The model under review builds one solid part; all positions refer to its coordinate system, in mm. Face numbers are marked on the shaded views. A direction names the side the tool comes from. Coordinates: 2 decimals unless noted, no trailing zeros. Write each loop counter-clockwise with the first axis right and the second up, starting at its lowest first coordinate (ties: lowest second). Pieces come first, ordered by that corner, then holes.
1) Add section B-B, the plane x = 0.5. State the section outline as (y, z) points.
2) For P1, Ø1.4, axis at x = 0.5, y = 12.5, coming from the +Z side; P2, Ø1, axis at y = 23.5, z = 0.5, coming from the +X side; P3, Ø1, axis at y = 29, z = 0, coming from the -X side; P4, Ø3, axis at x = 0, y = 1, coming from the -Z side, all flat-tipped, find the tip position at first contact; note any pin that passes through.
3) Add section C-C, the plane y = 2.5. State the section outline as (x, z) points, then the cut area to 3 significant figures.
4) Add section A-A, the plane y = 27.5. State the section outline as (x, z) points, then the cut area to 3 significant figures.
5) For line 1 (X direction, y = 24, z = 0); line 2 (Z direction, x = 1.25, y = 11), list the stretches that pass through material, from the lowest coordinate up.
6) Add section D-D, the plane x = 3.5. State the section outline as (y, z) points, then the cut area to 3 significant figures.
7) Machinability: for the marked faces 1, 2, 3 and 4, which of the approach directions +Z, -Z, +X, -X, +Y, -Y give a long, thin tool a straight path to every point of the face, cutting with its end or side? Answer none if there is none.
from build123d import *

# Parameters (mm, degrees)
EXTRUDE_THIN1_DEPTH      = 30.4
EXTRUDE_THIN1_DEPTH_BACK = 1.6
EXTRUDE_THIN2_DEPTH      = 12
EXTRUDE_THIN3_DEPTH      = 1


with BuildPart() as part:
    # Sketch1 → Extrude-Thin1 (new body, two sides)
    with BuildSketch(Plane(origin=(0, 0, 0), x_dir=(1, 0, 0), z_dir=(0, 1, 0))) as extrude_thin1_sk:
        with BuildLine():
            Line((1.35, -0.6), (-1.35, -0.6))
            ThreePointArc((-1.35, -0.6), (-1.456066017, -0.556066017), (-1.5, -0.45))
            Line((-1.5, -0.45), (-1.5, 0.45))
            ThreePointArc((-1.5, 0.45), (-1.456066017, 0.556066017), (-1.35, 0.6))
            Line((-1.35, 0.6), (1.35, 0.6))
            ThreePointArc((1.35, 0.6), (1.456066017, 0.556066017), (1.5, 0.45))
            Line((1.5, 0.45), (1.5, -0.45))
            ThreePointArc((1.5, -0.45), (1.456066017, -0.556066017), (1.35, -0.6))
        make_face()
        with BuildLine():
            Line((1.35, -0.5), (-1.35, -0.5))
            ThreePointArc((-1.35, -0.5), (-1.385355339, -0.485355339), (-1.4, -0.45))
            Line((-1.4, -0.45), (-1.4, 0.45))
            ThreePointArc((-1.4, 0.45), (-1.385355339, 0.485355339), (-1.35, 0.5))
            Line((-1.35, 0.5), (1.35, 0.5))
            ThreePointArc((1.35, 0.5), (1.385355339, 0.485355339), (1.4, 0.45))
            Line((1.4, 0.45), (1.4, -0.45))
            ThreePointArc((1.4, -0.45), (1.385355339, -0.485355339), (1.35, -0.5))
        make_face(mode=Mode.SUBTRACT)
    extrude(amount=EXTRUDE_THIN1_DEPTH)
    extrude(extrude_thin1_sk.sketch, amount=-EXTRUDE_THIN1_DEPTH_BACK)

    # Sketch2 → Extrude-Thin2 (add, symmetric)
    with BuildSketch(Plane(origin=(0, 14, 0), x_dir=(-1, 0, 0), z_dir=(0, 1, 0))):
        with BuildLine():
            Line((-1.55, -0.45), (-1.55, 0.45))
            ThreePointArc((-1.55, 0.45), (-1.491421356, 0.591421356), (-1.35, 0.65))
            Line((-1.35, 0.65), (1.35, 0.65))
            ThreePointArc((1.35, 0.65), (1.491421356, 0.591421356), (1.55, 0.45))
            Line((1.55, 0.45), (1.55, -0.45))
            ThreePointArc((1.55, -0.45), (1.491421356, -0.591421356), (1.35, -0.65))
            Line((1.35, -0.65), (-1.35, -0.65))
            ThreePointArc((-1.35, -0.65), (-1.491421356, -0.591421356), (-1.55, -0.45))
        make_face()
        with BuildLine():
            Line((-1.5, -0.45), (-1.5, 0.45))
            ThreePointArc((-1.5, 0.45), (-1.456066017, 0.556066017), (-1.35, 0.6))
            Line((-1.35, 0.6), (1.35, 0.6))
            ThreePointArc((1.35, 0.6), (1.456066017, 0.556066017), (1.5, 0.45))
            Line((1.5, 0.45), (1.5, -0.45))
            ThreePointArc((1.5, -0.45), (1.456066017, -0.556066017), (1.35, -0.6))
            Line((1.35, -0.6), (-1.35, -0.6))
            ThreePointArc((-1.35, -0.6), (-1.456066017, -0.556066017), (-1.5, -0.45))
        make_face(mode=Mode.SUBTRACT)
    extrude(amount=EXTRUDE_THIN2_DEPTH, both=True)

    # Sketch3 → Extrude-Thin3 (add)
    with BuildSketch(Plane.XZ.offset(0.5)):
        with BuildLine():
            Line((0, 0.6), (-0.75, 0.6))
            ThreePointArc((-0.75, 0.6), (-1.043338791, 0.837132251), (-0.872943663, 1.173650974))
            ThreePointArc((-0.872943663, 1.173650974), (2.074168878, 1.680733699), (4.9, 0.702324945))
            Line((4.9, 0.702324945), (5.733615576, 0.149979879))
            Line((5.733615576, 0.149979879), (5.678381069, 0.066618321))
            Line((5.678381069, 0.066618321), (4.844765493, 0.618963387))
            ThreePointArc((4.844765493, 0.618963387), (2.066031557, 1.581065329), (-0.831962442, 1.082433983))
            ThreePointArc((-0.831962442, 1.082433983), (-0.945559194, 0.858088167), (-0.75, 0.7))
            Line((-0.75, 0.7), (0, 0.7))
            Line((0, 0.7), (0, 0.6))
        make_face()
    extrude(amount=EXTRUDE_THIN3_DEPTH)


solid = part.part
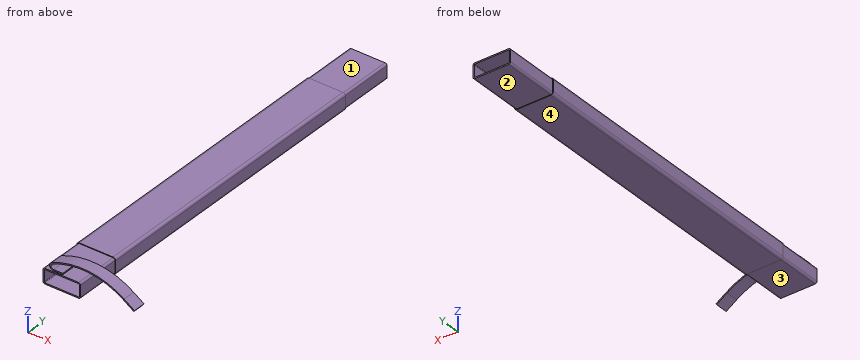
Geometry results:
1. outline: (-1.6, -0.6) - (2, -0.6) - (2, -0.65) - (26, -0.65) - (26, -0.6) - (30.4, -0.6) - (30.4, -0.5) - (-1.6, -0.5) - close; (-1.6, 0.5) - (30.4, 0.5) - (30.4, 0.6) - (26, 0.6) - (26, 0.65) - (2, 0.65) - (2, 0.6) - (-1.6, 0.6) - close; (-1.5, 1.5) - (-0.5, 1.5) - (-0.5, 1.6) - (-1.5, 1.6) - close
2. P1: stops at z = 0.65
2. P2: stops at x = 1.55
2. P3: stops at x = -1.5
2. P4: stops at z = -0.65
3. outline: (-1.55, -0.45) arc R0.2 ccw to (-1.35, -0.65) - (1.35, -0.65) arc R0.2 ccw to (1.55, -0.45) - (1.55, 0.45) arc R0.2 ccw to (1.35, 0.65) - (-1.35, 0.65) arc R0.2 ccw to (-1.55, 0.45) - close; hole (-1.4, -0.45) arc R0.05 ccw to (-1.35, -0.5) - (1.35, -0.5) arc R0.05 ccw to (1.4, -0.45) - (1.4, 0.45) arc R0.05 ccw to (1.35, 0.5) - (-1.35, 0.5) arc R0.05 ccw to (-1.4, 0.45) - close
3. area: 1.20 mm2
4. outline: (-1.5, -0.45) arc R0.15 ccw to (-1.35, -0.6) - (1.35, -0.6) arc R0.15 ccw to (1.5, -0.45) - (1.5, 0.45) arc R0.15 ccw to (1.35, 0.6) - (-1.35, 0.6) arc R0.15 ccw to (-1.5, 0.45) - close; hole (-1.4, -0.45) arc R0.05 ccw to (-1.35, -0.5) - (1.35, -0.5) arc R0.05 ccw to (1.4, -0.45) - (1.4, 0.45) arc R0.05 ccw to (1.35, 0.5) - (-1.35, 0.5) arc R0.05 ccw to (-1.4, 0.45) - close
4. area: 0.783 mm2
5. line 1: x = -1.55 to -1.4, 1.4 to 1.55
5. line 2: z = -0.65 to -0.5, 0.5 to 0.65
6. outline: (-1.5, 1.28) - (-0.5, 1.28) - (-0.5, 1.39) - (-1.5, 1.39) - close
6. area: 0.106 mm2
7. face 1: +Z, +X, -X, +Y
7. face 2: -Z, +X, -X, +Y
7. face 3: -Z, +X, -X, -Y
7. face 4: -Z, +X, -X, +Y, -Y
